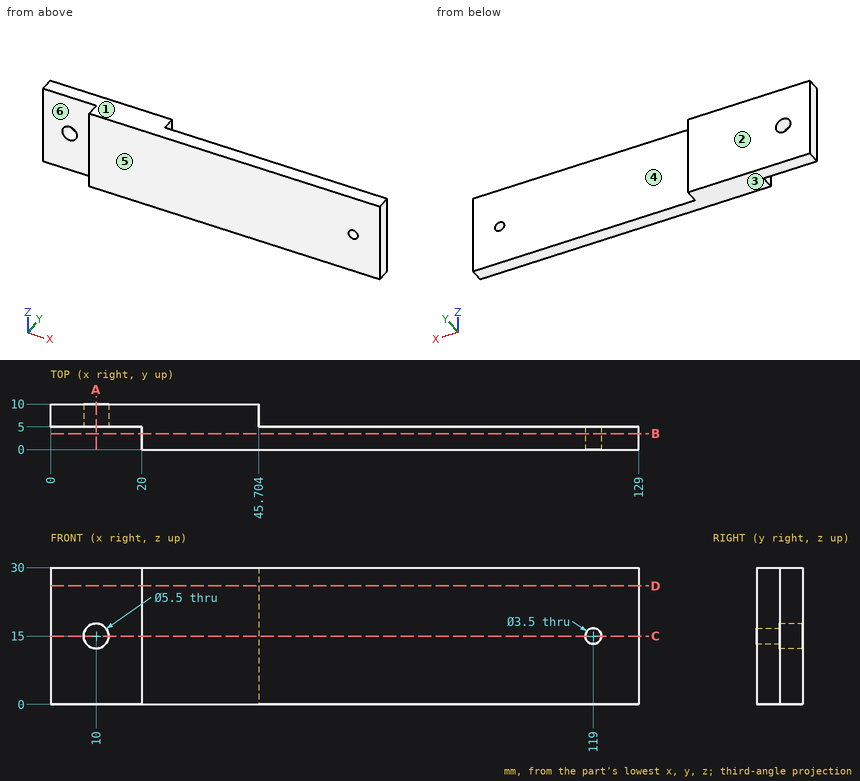
Design review of the part shown in the three views and the two pictorial views. Dimensions are in mm from the part's minimum x, y and z. A direction names the side the tool comes from. Coordinates: 2 decimals unless noted, no trailing zeros. Write each loop counter-clockwise with the first axis right and the second up, starting at its lowest first coordinate (ties: lowest second). Pieces come first, ordered by that corner, then holes.
1) We need section D-D on z = 26. State the section outline as (x, y) points (1 decimal).
2) We need section A-A on x = 10. State the section outline as (y, z) points.
3) Machinability: for the marked faces 4, 5 and 6, which of the approach directions +Z, -Z, +X, -X, +Y, -Y give a long, thin tool a straight path to every point of the face, cutting with its end or side? Answer none if there is none.
4) To check wall thickness, follow probe 1 along X at (y, z) = (2.9, 15); probe 2 along Z at (x, y) = (10, 7.25); probe 3 along Z at (x, y) = (119, 3.85). State the ranges of each line that lie inside material, in increasing order.
5) The part is to be moulded in two halves that separate along Z. For the marked faces 1, 2 and 3, say which applies: pulls with the +Z half, pulls with the -Z half, needs draft (parallel to the pull), parting line crosses it, or undercut.
6) Clearance check with flat-ended pins moving along their axes: pin 1 Ø5.5 at (x, z) = (119, 15) entering from +Y; pin 2 Ø1.5 at (y, z) = (7.5, 21.5) entering from +X; pin 3 Ø16 at (x, z) = (6, 10) entering from -Y. State where each tip first meets the part, or that it passes through.
7) We need section C-C on z = 15. Count the separate pieces of the cut face and the enclosed holes in it.
8) We need section B-B on y = 3.5. State the section outline as (x, z) points.
Answer list:
1. outline: (0, 5) - (20, 5) - (20, 0) - (129, 0) - (129, 5) - (45.7, 5) - (45.7, 10) - (0, 10) - close
2. outline: (5, 0) - (10, 0) - (10, 12.25) - (5, 12.25) - close; (5, 17.75) - (10, 17.75) - (10, 30) - (5, 30) - close
3. face 4: +Z, -Z, +X, +Y
3. face 5: +Z, -Z, +X, -X, -Y
3. face 6: +Z, -Z, -X, -Y
4. probe 1: x = 20 to 117.25, 120.75 to 129
4. probe 2: z = 0 to 12.25, 17.75 to 30
4. probe 3: z = 0 to 13.25, 16.75 to 30
5. face 1: pulls with the +Z half
5. face 2: needs draft
5. face 3: pulls with the -Z half
6. pin 1: stops at y = 5
6. pin 2: stops at x = 45.7
6. pin 3: stops at y = 5
7. separate pieces: 3
7. enclosed holes: 0
8. outline: (20, 0) - (129, 0) - (129, 30) - (20, 30) - close; hole circle Ø3.5 at (119, 15)
